from build123d import *

# Parameters (mm, degrees)
SKETCH_W        = 54.3
SKETCH_H        = 38
PAD_DEPTH       = 2
SKETCH001_W     = 54.3
SKETCH001_H     = 2
PAD001_DEPTH    = 22
SKETCH002_R     = 2.45
PAD002_DEPTH    = 5
SKETCH003_W     = 40
SKETCH003_H     = 22
PAD003_DEPTH    = 2
SKETCH004_W     = 40
SKETCH004_H     = 22
PAD004_DEPTH    = 2
SKETCH005_W     = 6.85
SKETCH005_H     = 15
PAD005_DEPTH    = 8
SKETCH006_R     = 1.4
POCKET_DEPTH    = 15
FILLET_R        = 3
FILLET001_R     = 2
SKETCH007_W     = 6.85
SKETCH007_H     = 25.8
PAD006_DEPTH    = 20
SKETCH008_R     = 1.4
POCKET001_DEPTH = 15
PAD007_DEPTH    = 2
SKETCH010_R     = 1.4
PAD008_DEPTH    = 2
SKETCH011_R     = 1.4
PAD009_DEPTH    = 2
SKETCH012_R     = 1.4
PAD010_DEPTH    = 5
SKETCH013_W     = 6.395784
SKETCH013_H     = 2
PAD011_DEPTH    = 5
CHAMFER_SIZE2   = 1.5
CHAMFER_SIZE    = 4


with BuildPart() as body:
    # Sketch → Pad (new body)
    with BuildSketch(Plane.XY):
        with Locations((27.15, 21)):
            Rectangle(SKETCH_W, SKETCH_H)
    extrude(amount=PAD_DEPTH)

    # Sketch001 → Pad001 (join)
    with BuildSketch(Plane.XY):
        with Locations((27.15, 1)):
            Rectangle(SKETCH001_W, SKETCH001_H)
    extrude(amount=PAD001_DEPTH)

    # Sketch002 → Pad002 (join)
    with BuildSketch(Plane.XZ):
        with Locations((37.25, 12)):
            Circle(SKETCH002_R)
    extrude(amount=PAD002_DEPTH)

    # Sketch003 (on Face2 of Pad002) → Pad003 (join)
    with BuildSketch(Plane(origin=(0, 0, 0), x_dir=(0, -1, 0), z_dir=(-1, 0, 0))):
        with Locations((-20, 11)):
            Rectangle(SKETCH003_W, SKETCH003_H)
    extrude(amount=PAD003_DEPTH)

    # Sketch004 (on Face3 of Pad003) → Pad004 (join)
    with BuildSketch(Plane.YZ.offset(54.3)):
        with Locations((20, 11)):
            Rectangle(SKETCH004_W, SKETCH004_H)
    extrude(amount=PAD004_DEPTH)

    # Sketch005 (on Face5 of Pad004) → Pad005 (join)
    with BuildSketch(Plane.XY.offset(2)):
        with Locations((50.875, 20.3)):
            Rectangle(SKETCH005_W, SKETCH005_H)
    extrude(amount=PAD005_DEPTH)

    # Sketch006 (on Face15 of Pad005) → Pocket (cut)
    with BuildSketch(Plane(origin=(0, 27.8, 0), x_dir=(-1, 0, 0), z_dir=(0, 1, 0))):
        with Locations((-51.3, 7)):
            Circle(SKETCH006_R)
    extrude(amount=-POCKET_DEPTH, mode=Mode.SUBTRACT)

    # Fillet
    fillet_edges = [body.edges().sort_by_distance(p)[0] for p in [
        (47.45, 20.3, 10),
    ]]
    fillet(fillet_edges, radius=FILLET_R)

    # Fillet001
    fillet001_edges = [body.edges().sort_by_distance(p)[0] for p in [
        (52.375, 12.8, 10),
    ]]
    fillet(fillet001_edges, radius=FILLET001_R)

    # Sketch007 (on Face5 of Fillet001) → Pad006 (join)
    with BuildSketch(Plane.XY.offset(2)):
        with Locations((3.425, 14.9)):
            Rectangle(SKETCH007_W, SKETCH007_H)
    extrude(amount=PAD006_DEPTH)

    # Sketch008 (on Face14 of Pad006) → Pocket001 (cut)
    with BuildSketch(Plane(origin=(0, 27.8, 0), x_dir=(-1, 0, 0), z_dir=(0, 1, 0))):
        with Locations((-3, 7)):
            Circle(SKETCH008_R)
        with Locations((-3, 17)):
            Circle(SKETCH008_R)
    extrude(amount=-POCKET001_DEPTH, mode=Mode.SUBTRACT)

    # Sketch009 (on Face21 of Pocket001) → Pad007 (join)
    with BuildSketch(Plane.XY.offset(22)):
        Polygon((54.3, 2), (54.3, 40), (56.3, 40), (56.3, 0), (-2, 0), (-2, 40), (6.85, 40), (6.85, 2), align=None)
    extrude(amount=PAD007_DEPTH)

    # Sketch010 (on Face22 of Pad007) → Pad008 (join)
    with BuildSketch(Plane.YZ.offset(6.85)):
        with BuildLine():
            Line((2, 24), (38, 24))
            Line((38, 29), (38, 24))
            ThreePointArc((38, 29), (37.326745, 31.511013), (35.487593, 33.348396))
            Line((35.487593, 33.348396), (9.497223, 48.331729))
            ThreePointArc((9.497223, 48.331729), (4.498612, 48.329325), (2, 44))
            Line((2, 44), (2, 24))
        make_face()
        with Locations((7, 44)):
            Circle(SKETCH010_R, mode=Mode.SUBTRACT)
        with Locations((32.980762, 29)):
            Circle(SKETCH010_R, mode=Mode.SUBTRACT)
    extrude(amount=-PAD008_DEPTH)

    # Sketch011 (on Face20 of Pad008) → Pad009 (join)
    with BuildSketch(Plane(origin=(54.3, 0, 0), x_dir=(0, -1, 0), z_dir=(-1, 0, 0))):
        with BuildLine():
            Line((-38, 24), (-38, 29))
            ThreePointArc((-35.487593, 33.348396), (-37.326745, 31.511013), (-38, 29))
            Line((-35.487593, 33.348396), (-9.497223, 48.331729))
            ThreePointArc((-2, 44), (-4.498612, 48.329325), (-9.497223, 48.331729))
            Line((-2, 44), (-2, 24))
            Line((-2, 24), (-38, 24))
        make_face()
        with Locations((-7, 44)):
            Circle(SKETCH011_R, mode=Mode.SUBTRACT)
        with Locations((-32.980762, 29)):
            Circle(SKETCH011_R, mode=Mode.SUBTRACT)
    extrude(amount=-PAD009_DEPTH)

    # Sketch012 (on Face35 of Pad009) → Pad010 (join)
    with BuildSketch(Plane.YZ.offset(6.85)):
        with BuildLine():
            Line((38, 29), (38, 24))
            Line((38, 24), (31.604216, 24))
            Line((30.473931, 24.651604), (31.604216, 24))
            Line((4.502799, 39.668258), (30.473931, 24.651604))
            ThreePointArc((9.497223, 48.331729), (2.668265, 46.497212), (4.502799, 39.668258))
            Line((9.497223, 48.331729), (35.487593, 33.348396))
            ThreePointArc((38, 29), (37.326745, 31.511013), (35.487593, 33.348396))
        make_face()
        with Locations((7, 44)):
            Circle(SKETCH012_R, mode=Mode.SUBTRACT)
        with Locations((32.980762, 29)):
            Circle(SKETCH012_R, mode=Mode.SUBTRACT)
    extrude(amount=PAD010_DEPTH)

    # Sketch013 (on Face22 of Pad010) → Pad011 (join)
    with BuildSketch(Plane.YZ.offset(6.85)):
        with Locations((34.802108, 23)):
            Rectangle(SKETCH013_W, SKETCH013_H)
    extrude(amount=PAD011_DEPTH)

    # Chamfer
    chamfer_edges = [body.edges().sort_by_distance(p)[0] for p in [
        (11.85, 34.802108, 22),
    ]]
    chamfer_side = body.faces().sort_by_distance((9.35, 34.802108, 22))[0]
    chamfer(chamfer_edges, length=CHAMFER_SIZE, length2=CHAMFER_SIZE2, reference=chamfer_side)


with BuildPart() as part_mirroring:
    # Part__Mirroring: instance of Body
    add(body.part.mirror(Plane(origin=(0, 0, 0), x_dir=(0, -1, 0), z_dir=(1, 0, 0))))


solid = part_mirroring.part
The listing builds one solid part. Answer for the finished solid, in the listing's coordinates (mm). A direction names the side the tool comes from. Coordinates: 2 decimals unless noted, no trailing zeros. Order: outer loops, then holes, each group sorted by start corner. A loop starts at its lowest first (then second) coordinate and runs counter-clockwise, first axis right, second up. Notation, with made-up numbers: M 55.5,14.5 L 100.5,14.5 A33 cw 100.5,47.5 Z; hole C 16.5,81.25 d11. An arc over 180 degrees is marked long. Use CSV: the item, a comma, the result in double quotes.
Q1. Section C-C (y = 3.5) is taken. Determine the outline of the cut face in (x, z).
Here are the results:
outline,"M -56.3,0 L 2,0 L 2,24 L -4.85,24 L -4.85,47.57 L -11.85,47.57 L -11.85,40.43 L -6.85,40.43 L -6.85,2 L -54.3,2 L -54.3,47.57 L -56.3,47.57 Z"
Q2. Section A-A (z = 17) is taken. Determine the outline of the cut face in (x, y).
Here are the results:
outline,"M -56.3,0 L 2,0 L 2,40 L 0,40 L 0,27.8 L -1.6,27.8 L -1.6,12.8 L -4.4,12.8 L -4.4,27.8 L -6.85,27.8 L -6.85,2 L -54.3,2 L -54.3,40 L -56.3,40 Z"
Q3. Section D-D (z = 26.5) is taken. Determine the outline of the cut face in (x, y), then the cut area to 3 significant figures.
Here are the results:
outline,"M -56.3,2 L -54.3,2 L -54.3,38 L -56.3,38 Z; M -11.85,27.28 L -6.85,27.28 L -6.85,2 L -4.85,2 L -4.85,38 L -11.85,38 Z"
area,"198 mm2"
Q4. Straight lines are drawn through the part: L1, parallel to Z at x = -3, y = 21; L2, parallel to X at y = 6.5, z = 8; L3, parallel to Z at x = -8.5, y = 4.5. For each, find the intervals that lie inside material, in ascending order.
Here are the results:
L1,"0 to 5.6, 8.4 to 15.6, 18.4 to 24"
L2,"-56.3 to -54.3, -6.85 to 2"
L3,"0 to 2, 39.67 to 48.33"
Q5. Determine the mould class of faces 5 (the flat face through (-51, 27.8, 5)), 6 (the flat face through (-47.45, 21, 4)), 7 (the cylindrical face through (-8.3, 32.8, 30.39)) for opening direction Y: pulls with the +Y half, pulls with the -Y half, needs draft (parallel to the pull), parting line crosses it, or undercut.
Here are the results:
face 5,"pulls with the +Y half"
face 6,"needs draft"
face 7,"undercut"
Q6. Given pin 1 Ø2.5 at (x, z) = (-53, 4.5) entering from -Y; pin 2 Ø5 at (y, z) = (4.5, 40) entering from +X; pin 3 Ø3 at (x, z) = (-3, 17) entering from +Y, each flat-ended and moving along its own axis, determine where each tip first touches the part or whether it passes through.
Here are the results:
pin 1,"y = 0"
pin 2,"x = -4.85"
pin 3,"y = 27.8"
Q7. Section B-B (x = -15) is taken. Determine the outline of the cut face in (y, z), then the cut area to 3 significant figures.
Here are the results:
outline,"M 0,0 L 40,0 L 40,2 L 2,2 L 2,24 L 0,24 Z"
area,"124 mm2"
Q8. A tool of negligible diameter and unlimited length cuts with its end or side. For faces 1 (the flat face through (-6.85, 39, 23)), 2 (the flat face through (-6, 2, 34)), 3 (the cylindrical face through (-53.3, 13.4, 9.43)), 4 (the flat face through (-3, 12.8, 7)), from which of +Z, -Z, +X, -X, +Y, -Y can it reach the whole face along a straight path? Write none if from no direction.
Here are the results:
face 1,"+Z, +Y"
face 2,"+Z, +X, -X, -Y"
face 3,"+Z"
face 4,"+Y"
